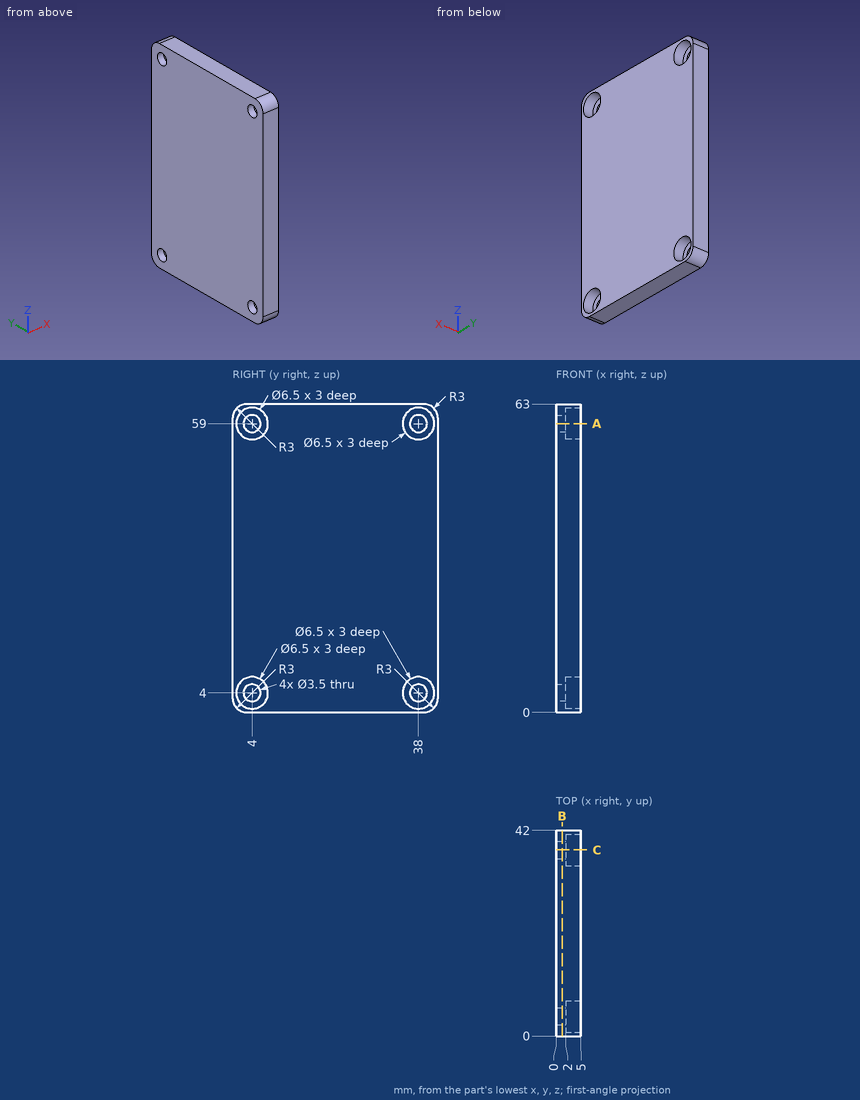
Part print with two shaded views. Sizes in mm from the minimum x, y, z corner. Give positions to 0.01 mm unless a question says otherwise; leave off trailing zeros. Loops run counter-clockwise (first coordinate to the right, second up) from the corner with the lowest first, then second, coordinate; pieces in that order, holes last. Notation, with made-up numbers: (-37, 34.25) - (5, 34.25) arc R27 cw to (5, 70.25) - close; hole circle Ø9 at (25.5, 51.25). An arc over 180 degrees is marked (long way). Put each result on its own line as item: value.
Q1. Slice it at C-C (y = 38). Give the cut face in (x, z).
Filled in:
outline: (0, 0) - (5, 0) - (5, 0.75) - (2, 0.75) - (2, 2.25) - (0, 2.25) - close; (0, 5.75) - (2, 5.75) - (2, 7.25) - (5, 7.25) - (5, 55.75) - (2, 55.75) - (2, 57.25) - (0, 57.25) - close; (0, 60.75) - (2, 60.75) - (2, 62.25) - (5, 62.25) - (5, 63) - (0, 63) - close
Q2. Probe line 1 along Y through (x, z) = (3.4, 4); line 2 along Y through (x, z) = (1.05, 59); line 3 along Z through (x, y) = (1.4, 39). List the from-to ranges inside material, lowest first.
Filled in:
line 1: y = 0 to 0.75, 7.25 to 34.75, 41.25 to 42
line 2: y = 0 to 2.25, 5.75 to 36.25, 39.75 to 42
line 3: z = 0 to 2.56, 5.44 to 57.56, 60.44 to 63
Q3. Slice it at A-A (z = 59). Give the cut face in (x, y).
Filled in:
outline: (0, 0) - (5, 0) - (5, 0.75) - (2, 0.75) - (2, 2.25) - (0, 2.25) - close; (0, 5.75) - (2, 5.75) - (2, 7.25) - (5, 7.25) - (5, 34.75) - (2, 34.75) - (2, 36.25) - (0, 36.25) - close; (0, 39.75) - (2, 39.75) - (2, 41.25) - (5, 41.25) - (5, 42) - (0, 42) - close
Q4. Slice it at B-B (x = 1.25). Give the cut face in (y, z), plus the area to 3 significant figures.
Filled in:
outline: (0, 3) arc R3 ccw to (3, 0) - (39, 0) arc R3 ccw to (42, 3) - (42, 60) arc R3 ccw to (39, 63) - (3, 63) arc R3 ccw to (0, 60) - close; hole circle Ø3.5 at (4, 4); hole circle Ø3.5 at (4, 59); hole circle Ø3.5 at (38, 4); hole circle Ø3.5 at (38, 59)
area: 2,600 mm²
Q5. Flat gauge pin, fed straight in: pin 1 (3 mm diameter, centred on y = 37.5, z = 4.5, fed in from +X). Where does the tip first touch, or does it go through?
Filled in:
pin 1: stops at x = 2
